The model under review builds one solid part; all positions refer to its coordinate system, in mm. A direction names the side the tool comes from. Coordinates: 2 decimals unless noted, no trailing zeros. Write each loop counter-clockwise with the first axis right and the second up, starting at its lowest first coordinate (ties: lowest second). Pieces come first, ordered by that corner, then holes. Notation, with made-up numbers: (-32, 37) - (-11, 37) arc R30 ccw to (-11, 70) - close; hole circle Ø3 at (-38, 13.25). An arc over 180 degrees is marked (long way). Return JSON: item names as keys, results as strings. Group by question number.
(1) For pin 1 Ø1.5 at (x, z) = (0, -4) entering from -Y; pin 2 Ø7.5 at (x, y) = (-5.5, -26) entering from -Z; pin 3 Ø2.5 at (x, z) = (-1, 1.5) entering from +Y, all flat-tipped, find the tip position at first contact; note any pin that passes through.
(2) To check wall thickness, follow L1, parallel to X at y = -2, z = 0.5; L2, parallel to Z at x = 1.5, y = -11; L3, parallel to Y at x = -0.25, z = 0.5. State the ranges of each line that lie inside material, in increasing order. Write a range as from..to.
(3) Draft analysis for pull direction Y (two halves, no side actions). For faces 5 (the face through (-1, -11, 0)), 6 (the face through (6.933, -39.439, 2.396)), 7 (the face through (-5.335, -0.384, 1.479)), 8 (the face through (-5.75, -26.92, 0.86)), state which applies: released by +Y, released by -Y, zero draft, split by the parting line, or undercut.
(4) Tool access review of faces 1 (the face through (-6, -17.059, 0.9)), 2 (the face through (8.937, -10.859, 0.601)), 3 (the face through (0, -5.059, 1)), 4 (the face through (-0.3, -37.3, -6.5)): name each direction out of +Z, -Z, +X, -X, +Y, -Y from which nothing blocks a thin tool from reaching the whole face with its end or side.
(5) We need section B-B on z = 2.5. State the section outline as (x, y) points, then the cut area to 3 significant figures.
```python
from build123d import *
from OCP.BRepFilletAPI import BRepFilletAPI_MakeChamfer

# Parameters (mm, degrees)
SKETCH1_R           = 2.25
BOSS_EXTRUDE1_DEPTH = 3
BOSS_EXTRUDE2_DEPTH = 3
BOSS_EXTRUDE3_DEPTH = 7.5
CHAMFER1_SIZE       = 7
CHAMFER1_SIZE2      = 4.041451884
CUT_EXTRUDE1_DEPTH  = 47.864827652
FILLET1_R           = 3
CHAMFER2_SIZE       = 2
CHAMFER2_SIZE2      = 2.328114762
CHAMFER3_SIZE       = 5
CHAMFER3_SIZE2      = 1.819851171
CUT_EXTRUDE2_DEPTH  = 47.864827652
FILLET2_R           = 2


with BuildPart() as part:
    # Sketch1 → Boss-Extrude1 (new body)
    with BuildSketch(Plane.XY):
        Polygon((2.018448149, -5.059414071), (-2.981551851, -5.059414071), (-2.981551851, 4.940585929), (-12.981551851, 4.940585929), (-12.981551851, -7.059414071), (12.018448149, -7.059414071), (12.018448149, 4.940585929), (2.018448149, 4.940585929), align=None)
        with Locations((6.518448149, -1.059414071)):
            Circle(SKETCH1_R, mode=Mode.SUBTRACT)
        with Locations((-7.481551851, -1.059414071)):
            Circle(SKETCH1_R, mode=Mode.SUBTRACT)
    extrude(amount=BOSS_EXTRUDE1_DEPTH)

    # Sketch2 → Boss-Extrude2 (add, through all)
    with BuildSketch(Plane.XY.offset(3)):
        Polygon((-12.981551851, -7.059414071), (-8.981551851, -37.059414071), (8.018448149, -37.059414071), (12.018448149, -7.059414071), align=None)
    extrude(amount=-BOSS_EXTRUDE2_DEPTH)

    # Sketch4 → Boss-Extrude3 (add)
    with BuildSketch(Plane.XZ.offset(37.059414071)):
        with BuildLine():
            Line((-8.981551851, 2), (-8.981551851, 3))
            Line((-8.981551851, 3), (8.018448149, 3))
            Line((8.018448149, 3), (8.018448149, 2))
            ThreePointArc((8.018448149, 2), (-0.481551851, -6.5), (-8.981551851, 2))
        make_face()
    extrude(amount=BOSS_EXTRUDE3_DEPTH)

    # Chamfer1: one chamfer whose edges measure the first distance from different faces: ONE call of the kernel's chamfer builder (chamfer() names one face for all edges)
    chamfer1_edges_1 = [part.edges().sort_by_distance(p)[0] for p in [
        (-0.481551851, -44.559414071, -6.5),
    ]]
    chamfer1_side_1 = [part.faces().sort_by_distance(p)[0] for p in [
        (-0.481551851, -40.809414071, -6.5),
    ]]
    chamfer1_edges_2 = [part.edges().sort_by_distance(p)[0] for p in [
        (8.018448149, -44.559414071, 2.5),
    ]]
    chamfer1_side_2 = [part.faces().sort_by_distance(p)[0] for p in [
        (8.018448149, -40.809414071, 2.5),
    ]]
    chamfer1_edges_3 = [part.edges().sort_by_distance(p)[0] for p in [
        (-8.981551851, -44.559414071, 2.5),
    ]]
    chamfer1_side_3 = [part.faces().sort_by_distance(p)[0] for p in [
        (-8.981551851, -40.809414071, 2.5),
    ]]
    chamfer1 = BRepFilletAPI_MakeChamfer(part.part.solid().wrapped)
    for e in chamfer1_edges_1:
        chamfer1.Add(CHAMFER1_SIZE, CHAMFER1_SIZE2, e.wrapped, chamfer1_side_1[0].wrapped)  # the first distance lies on this face
    for e in chamfer1_edges_2:
        chamfer1.Add(CHAMFER1_SIZE, CHAMFER1_SIZE2, e.wrapped, chamfer1_side_2[0].wrapped)  # the first distance lies on this face
    for e in chamfer1_edges_3:
        chamfer1.Add(CHAMFER1_SIZE, CHAMFER1_SIZE2, e.wrapped, chamfer1_side_3[0].wrapped)  # the first distance lies on this face
    add(Compound.cast(chamfer1.Shape()), mode=Mode.REPLACE)

    # Sketch5 → Cut-Extrude1 (cut, through all)
    with BuildSketch(Plane(origin=(0, 0, 0), x_dir=(-1, 0, 0), z_dir=(0, 0, -1))):
        Polygon((6.648218517, -37.059414071), (6.648218517, -17.059414071), (11.648218517, -17.059414071), (8.981551851, -37.059414071), align=None)
        Polygon((-10.685114816, -17.059414071), (-8.018448149, -37.059414071), (-5.685114816, -37.059414071), (-5.685114816, -17.059414071), align=None)
    extrude(amount=-CUT_EXTRUDE1_DEPTH, mode=Mode.SUBTRACT)

    # Fillet1
    fillet1_edges = [part.edges().sort_by_distance(p)[0] for p in [
        (5.685114816, -27.059414071, 0),
        (-6.648218517, -27.059414071, 0),
    ]]
    fillet(fillet1_edges, radius=FILLET1_R - 0.0001)  # a hair under: the kernel refuses the full size

    # Chamfer2: one chamfer whose edges measure the first distance from different faces: ONE call of the kernel's chamfer builder (chamfer() names one face for all edges)
    chamfer2_edges_1 = [part.edges().sort_by_distance(p)[0] for p in [
        (2.018448149, 4.940585929, 1.5),
        (12.018448149, 4.940585929, 1.5),
        (-12.981551851, 4.940585929, 1.5),
        (-2.981551851, 4.940585929, 1.5),
    ]]
    chamfer2_edges_2 = [part.edges().sort_by_distance(p)[0] for p in [
        (-11.648218517, -17.059414071, 1.5),
    ]]
    chamfer2_side_2 = [part.faces().sort_by_distance(p)[0] for p in [
        (-12.314885184, -12.059414071, 1.5),
    ]]
    chamfer2_edges_3 = [part.edges().sort_by_distance(p)[0] for p in [
        (10.685114816, -17.059414071, 1.5),
    ]]
    chamfer2_side_3 = [part.faces().sort_by_distance(p)[0] for p in [
        (7.823515647, -17.059414071, 1.405334343),
    ]]
    chamfer2 = BRepFilletAPI_MakeChamfer(part.part.solid().wrapped)
    for e in chamfer2_edges_1:
        chamfer2.Add(CHAMFER2_SIZE, e.wrapped)
    for e in chamfer2_edges_2:
        chamfer2.Add(CHAMFER2_SIZE, CHAMFER2_SIZE2, e.wrapped, chamfer2_side_2[0].wrapped)  # the first distance lies on this face
    for e in chamfer2_edges_3:
        chamfer2.Add(CHAMFER2_SIZE, CHAMFER2_SIZE2, e.wrapped, chamfer2_side_3[0].wrapped)  # the first distance lies on this face
    add(Compound.cast(chamfer2.Shape()), mode=Mode.REPLACE)

    # Chamfer3
    chamfer3_edges = [part.edges().sort_by_distance(p)[0] for p in [
        (-0.481551851, -44.559414071, 3),
    ]]
    chamfer3_side = [part.faces().sort_by_distance(p)[0] for p in [
        (-0.481914427, -17.452973587, 3),
    ]]
    chamfer(chamfer3_edges, length=CHAMFER3_SIZE, length2=CHAMFER3_SIZE2, reference=chamfer3_side[0])

    # Sketch6 → Cut-Extrude2 (cut, through all)
    with BuildSketch(Plane(origin=(0, 0, 0), x_dir=(-1, 0, 0), z_dir=(0, 0, -1))):
        Polygon((-5.685114816, -17.059414071), (-12.018448149, -7.059414071), (-10.992807124, -14.751721764), (-8.685114816, -17.059414071), align=None)
        Polygon((12.981551851, -7.059414071), (6.648218517, -17.059414071), (9.320103756, -17.059414071), (11.912545957, -15.07695827), align=None)
    extrude(amount=-CUT_EXTRUDE2_DEPTH, mode=Mode.SUBTRACT)

    # Fillet2
    fillet2_edges = [part.edges().sort_by_distance(p)[0] for p in [
        (8.851781483, -12.059414071, 0),
        (-9.814885184, -12.059414071, 0),
    ]]
    fillet(fillet2_edges, radius=FILLET2_R)


solid = part.part
```
Ans:
{
 "1": {"pin 1": "y = -43.16", "pin 2": "z = 0", "pin 3": "y = -5.06"},
 "2": {"L1": "-12.98..-9.53, -5.44..-2.98, 2.02..4.47, 8.56..12.02", "L2": "0..3", "L3": "-44.56..-5.06"},
 "3": {"face 5": "zero draft", "face 6": "released by -Y", "face 7": "undercut", "face 8": "undercut"},
 "4": {"face 1": "-Z, -X", "face 2": "-Z, +X", "face 3": "+Z, -Z, +Y", "face 4": "-Z, -Y"},
 "5": {"outline": "(-12.98, -7.06) - (-6.65, -17.06) - (-6.61, -17.06) - (-6.61, -37.06) - (-8.98, -37.06) - (-8.98, -37.56) - (-7.03, -40.93) - (6.07, -40.93) - (8.02, -37.56) - (8.02, -37.06) - (5.64, -37.06) - (5.64, -17.06) - (5.69, -17.06) - (12.02, -7.06) - (12.02, 2.94) - (10.02, 4.94) - (4.02, 4.94) - (2.02, 2.94) - (2.02, -5.06) - (-2.98, -5.06) - (-2.98, 2.94) - (-4.98, 4.94) - (-10.98, 4.94) - (-12.98, 2.94) - close; hole circle Ø4.5 at (-7.48, -1.06); hole circle Ø4.5 at (6.52, -1.06)", "area": "701 mm²"}
}
